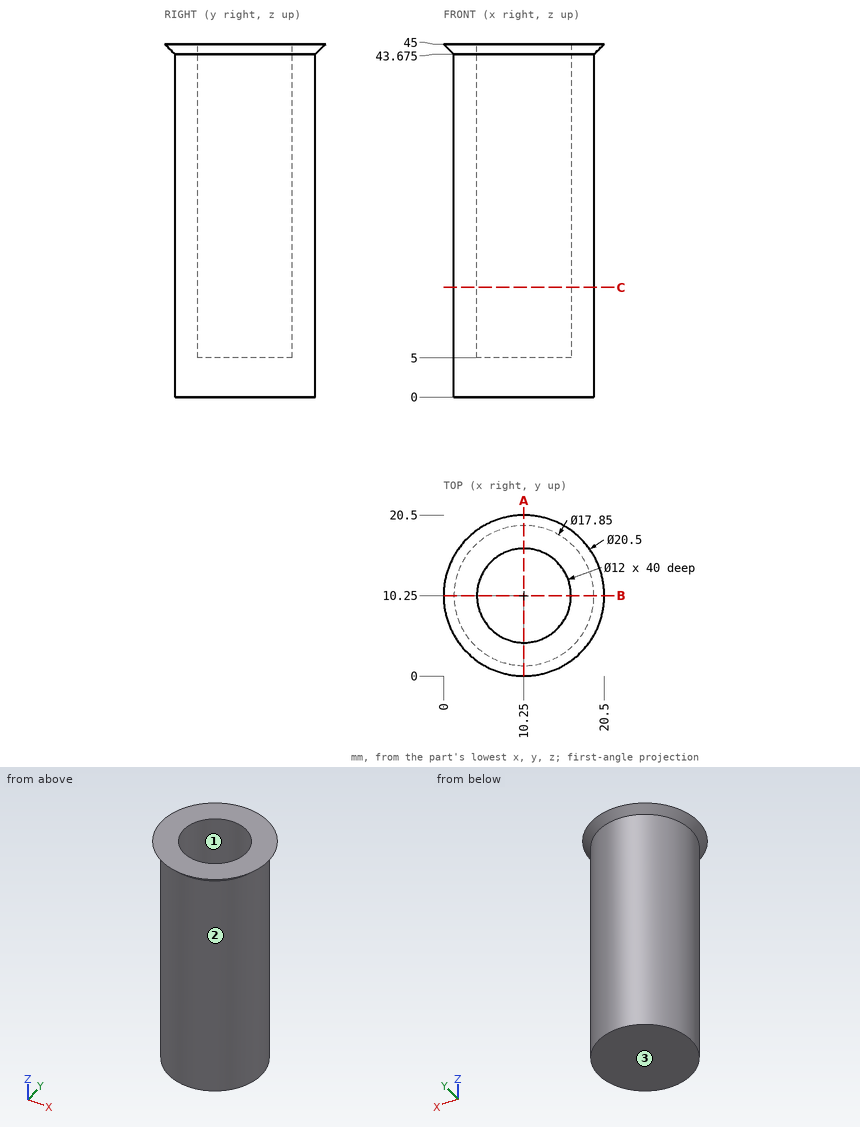
Answer from the drawing. Dimensions are ordinates in mm from the lowest x, y and z of the part. Round coordinates to 2 decimals unless told otherwise and drop trailing zeros. Loops run counter-clockwise (first coordinate to the right, second up) from the corner with the lowest first, then second, coordinate; pieces in that order, holes last.
1) A cutting plane is placed at C-C on z = 14. Determine the outline of the cut face in (x, y) (3 decimals), plus the area to 3 significant figures.
Outcome:
outline: circle Ø17.85 at (10.25, 10.25); hole circle Ø12 at (10.25, 10.25)
area: 137 mm2
2) Consider line 1 (Y direction, x = 10.25, z = 20.5) (3 decimals); line 2 (X direction, y = 10.5, z = 11); line 3 (Z direction, x = 5.25, y = 11.5). Determine where each line is inside the solid, lowest interval first.
Outcome:
line 1: y = 1.325 to 4.25, 16.25 to 19.175
line 2: x = 1.33 to 4.26, 16.24 to 19.17
line 3: z = 0 to 5
3) A cutting plane is placed at A-A on x = 10.25. Determine the outline of the cut face in (y, z) (3 decimals).
Outcome:
outline: (0, 45) - (1.325, 43.675) - (1.325, 0) - (19.175, 0) - (19.175, 43.675) - (20.5, 45) - (16.25, 45) - (16.25, 5) - (4.25, 5) - (4.25, 45) - close
4) For a pull along X with two mould halves and no side action, classify the marked faces 1, 2 and 3 as released by +X, released by -X, zero draft, split by the parting line, or undercut.
Outcome:
face 1: undercut
face 2: split by the parting line
face 3: zero draft
5) Given P1, Ø2, axis at x = 6, y = 7.5, coming from the +Z side; P2, Ø1.5, axis at y = 5.5, z = 9.5, coming from the +X side; P3, Ø2, axis at y = 14.5, z = 27, coming from the -X side; P4, Ø3, axis at x = 5, z = 4.5, coming from the -Y side, each flat-ended and moving along its own axis, determine where each tip first touches the part or whether it passes through.
Outcome:
P1: stops at z = 45
P2: stops at x = 18.23
P3: stops at x = 1.94
P4: stops at y = 2.15
